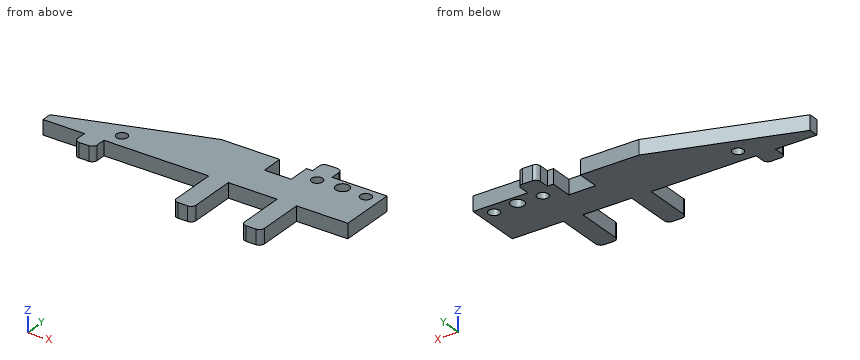
Autodesk Inventor part; units mm, degrees
ref_plane "YZ Plane" through (0, 0, 0) normal (1, 0, 0) x (0, 1, 0)
ref_plane "XZ Plane" through (0, 0, 0) normal (0, 1, 0) x (-1, 0, 0)
ref_plane "XY Plane" through (0, 0, 0) normal (0, 0, 1) x (1, 0, 0)
sketch "Sketch1" plane through (0, 0, 0) normal (0, 0, 1) x (1, 0, 0)
  line L0 (0, 4) -> (0, 0)
  line L1 (0, 0) -> (125, 0)
  line L2 (125, 0) -> (125, 23)
  line L3 (57, 23) -> (0, 4)
  line L4 (81, 23) -> (81, 14)
  line L5 (81, 14) -> (92, 14)
  line L6 (92, 14) -> (92, 23)
  line L7 (125, 23) -> (92, 23)
  line L8 (81, 23) -> (57, 23)
  circle A0 centre (99.5, 18.5) radius 2.25
  circle A1 centre (119.5, 18.5) radius 2.25
  circle A2 centre (28.2, 6) radius 2.25
  circle A3 centre (28.2, 6) radius 4.5 construction
  point P0 (92, 18.5)
  dimension "d0" = 4
  dimension "d1" = 125
  dimension "d2" = 9
  dimension "d3" = 11
  dimension "d4" = 33
  dimension "d5" = 24
  dimension "d6" = 23
  dimension "d7" = 4.5
  dimension "d8" = 4.5
  dimension "d9" = 5.5
  dimension "d10" = 20
  dimension "d11" = 4.5
  dimension "d12" = 9
  dimension "d13" = 6
  dimension "d14" = 28.2
extrude "Extrusion1" add sketch "Sketch1" along normal blind 6
sketch "Sketch2" plane through (0, 0, 6) normal (0, 0, 1) x (1, 0, 0)
  line L0 (0, 0) -> (125, 0)
  line L1 (125, 0) -> (125, 23)
  line L2 (125, 23) -> (92, 23)
  line L3 (17, 0) -> (25, 0)
  line L4 (25, 0) -> (25, -4)
  line L5 (23, -6) -> (19, -6)
  line L6 (17, -4) -> (17, 0)
  line L7 (96, 0) -> (104, 0)
  line L8 (104, 0) -> (104, -19)
  line L9 (102, -21) -> (98, -21)
  line L10 (96, -19) -> (96, 0)
  line L11 (68, 0) -> (76, 0)
  line L12 (76, 0) -> (76, -19)
  line L13 (74, -21) -> (70, -21)
  line L14 (68, -19) -> (68, 0)
  line L15 (94.5, 23) -> (102.5, 23)
  line L16 (102.5, 23) -> (102.5, 27)
  line L17 (100.5, 29) -> (96.5, 29)
  line L18 (94.5, 27) -> (94.5, 23)
  arc A0 (17, -4) -> (19, -6) centre (19, -4) ccw
  arc A1 (23, -6) -> (25, -4) centre (23, -4) ccw
  arc A2 (96, -19) -> (98, -21) centre (98, -19) ccw
  arc A3 (102, -21) -> (104, -19) centre (102, -19) ccw
  arc A4 (68, -19) -> (70, -21) centre (70, -19) ccw
  arc A5 (74, -21) -> (76, -19) centre (74, -19) ccw
  arc A6 (96.5, 29) -> (94.5, 27) centre (96.5, 27) ccw
  arc A7 (102.5, 27) -> (100.5, 29) centre (100.5, 27) ccw
  dimension "d17" = 2
  dimension "d18" = 17
  dimension "d20" = 8
  dimension "d21" = 8
  dimension "d22" = 8
  dimension "d24" = 6
  dimension "d25" = 43
  dimension "d26" = 20
  dimension "d29" = 8
  dimension "d32" = 22.5
  dimension "d40" = 6
  dimension "d41" = 2
  dimension "d42" = 2
  dimension "d45" = 21
sketch "Sketch3" plane through (0, 0, 6) normal (0, 0, 1) x (1, 0, 0)
  circle A0 centre (119.5, 18.5) radius 2.25
  circle A1 centre (109.5, 19.099) radius 2.75
  circle A2 centre (86.5, 19.099) radius 7.5 construction
  dimension "d35" = 5.5
  dimension "d36" = 15
  dimension "d37" = 10
extrude "Extrusion3" cut sketch "Sketch3" against normal blind 6 contours A1
extrude "Extrusion4" add sketch "Sketch2" against normal blind 6
properties part number "x_motor_upper_nut_stop"
CAD build for the part. Positions are in the model's coordinates, mm. Coordinates: 2 decimals unless noted, no trailing zeros. Write each loop counter-clockwise with the first axis right and the second up, starting at its lowest first coordinate (ties: lowest second). Pieces come first, ordered by that corner, then holes. Notation, with made-up numbers: M 49,-37 L 96,-37 A17 cw 96,-21 Z; hole C 6.25,3 d2. An arc over 180 degrees is marked long. Answer as a JSON object with one key per item and string values. Group by question number.
1) Saw through at B-B (x = 28.2). Write the cut outline in (y, z), plus the area to 3 significant figures.
2) Saw through at A-A (y = 6). Write the cut outline in (x, z).
3) Pin check, flat tips, straight feed: pin 1 Ø1.2 at (x, z) = (92.5, 3.5) entering from +Y; pin 2 Ø3 at (x, z) = (116, 4) entering from -Y; pin 3 Ø3 at (y, z) = (-12.5, 1.5) entering from -X; pin 4 Ø10 at (x, y) = (102.5, 17.5) entering from -Z. Stop position of each tip, or through.
4) Saw through at C-C (z = 2.45). Give the number of separate pieces and of enclosed holes in the cut face, plus the area to 3 significant figures.
5) Wall check: line 1 (Y direction, x = 109.5, z = 1.55); line 2 (X direction, y = -17, z = 5.25); line 3 (Y direction, x = 99.5, z = 2.8). Give the ranges that are in metal, low to high. Write a range as from..to.
6) Saw through at D-D (x = 60). Write the cut outline in (y, z), plus the area to 3 significant figures.
Values follow:
{
 "1": {"outline": "M 0,0 L 3.75,0 L 3.75,6 L 0,6 Z; M 8.25,0 L 13.4,0 L 13.4,6 L 8.25,6 Z", "area": "53.4 mm2"},
 "2": {"outline": "M 6,0 L 25.95,0 L 25.95,6 L 6,6 Z; M 30.45,0 L 125,0 L 125,6 L 30.45,6 Z"},
 "3": {"pin 1": "stops at y = 23", "pin 2": "stops at y = 0", "pin 3": "stops at x = 68", "pin 4": "stops at z = 0"},
 "4": {"separate pieces": "1", "enclosed holes": "4", "area": "2,590 mm2"},
 "5": {"line 1": "y = 0..16.35, 21.85..23", "line 2": "x = 68..76, 96..104", "line 3": "y = -21..16.25, 20.75..29"},
 "6": {"outline": "M 0,0 L 23,0 L 23,6 L 0,6 Z", "area": "138 mm2"}
}
